Autodesk Inventor part; units mm, degrees
ref_plane "YZ Plane" through (0, 0, 0) normal (1, 0, 0) x (0, 1, 0)
ref_plane "XZ Plane" through (0, 0, 0) normal (0, 1, 0) x (-1, 0, 0)
ref_plane "XY Plane" through (0, 0, 0) normal (0, 0, 1) x (1, 0, 0)
sketch "Sketch1" plane through (0, 0, 0) normal (0, 1, 0) x (-1, 0, 0)
  line L0 (-15, 20.25) -> (15, 20.25)
  line L1 (15, 20.25) -> (15, -20.25)
  line L2 (15, -20.25) -> (-15, -20.25)
  line L3 (-15, -20.25) -> (-15, 20.25)
  line L4 (-15, 20.25) -> (15, -20.25) construction
  line L5 (15, 20.25) -> (-15, -20.25) construction
  point P0 (0, 0)
  dimension "d0" = 40.5
  dimension "d1" = 30
extrude "Plate1" add sketch "Sketch1" along normal blind 1.5
sketch "Sketch2" plane through (-15, 0, -21.75) normal (0, 0, 1) x (1, 0, 0)
  line L0 (30, 0) -> (0, 0)
  line L1 (0, 0) -> (0, 35.9)
  line L2 (0, 35.9) -> (30, 35.9)
  line L3 (30, 35.9) -> (30, 0)
edge flange "Flange1" height 35.9 angle 90 thickness 1.5 bend radius 0.31 thickness toward (0, 0, 1) relief tear relief width 1.5 relief depth 0.75 corner gap 0.31 corner form 0 edges at (0, 1.5, -20.25) (0, 1.5, 20.25) wall of the first edge with corners at (15, 0, -21.75) (-15, 0, -21.75) (-15, 35.9, -21.75) (15, 35.9, -21.75)
bend "Bend1"
corner "Corner1"
sketch "Sketch3" plane through (0, 1.5, 0) normal (0, 1, 0) x (1, 0, 0)
  circle A0 centre (7, 0) radius 0.7835
  circle A1 centre (0, -7) radius 0.7835
  circle A2 centre (-7, 0) radius 0.7835
  circle A3 centre (0, 7) radius 0.7835
  point P0 (0, 0)
hole "Hole1" at (0, 1.5, 7) at (7, 1.5, 0) at (-7, 1.5, 0) at (0, 1.5, -7) direction (0, -1, 0) diameter 2.1 depth 1.5
sketch "Sketch26" plane through (-15, 35.9, 21.75) normal (0, 0, 1) x (1, 0, 0)
  line L0 (30, 9.1) -> (25, 9.1)
  line L1 (25, 9.1) -> (25, -25.9)
  line L2 (25, -25.9) -> (30, -25.9)
  line L3 (30, -25.9) -> (30, 9.1)
  line L4 (0, 9.1) -> (5, 9.1)
  line L5 (5, 9.1) -> (5, -25.9)
  line L6 (5, -25.9) -> (0, -25.9)
  line L7 (0, -25.9) -> (0, 9.1)
  point P0 (15, -35.9)
  dimension "d91" = 35
  dimension "d92" = 5
  dimension "d93" = 10
  dimension "d94" = 10
  dimension "d95" = 5
  dimension "d96" = 35
  dimension "d97" = 10
  dimension "d98" = 10
extrude "Cut11" cut sketch "Sketch26" against normal blind 1.5
fillet "Corner Round1" radius 5 1 edges at (-15, 10, 21)
fillet "Corner Round2" radius 5 1 edges at (15, 10, 21)
mirror "Mirror1" about plane through (0, 0, 0) normal (0, 0, 1) of "Cut11"
fillet "Corner Round3" radius 5 1 edges at (-15, 10, -21)
fillet "Corner Round4" radius 5 1 edges at (15, 10, -21)
fillet "Corner Round5" radius 1 4 edges at (10, 35.9, -21) (10, 35.9, 21) (-10, 35.9, 21) (-10, 35.9, -21)
sketch "Sketch31" plane through (-15, 1.81, 21.75) normal (0, 0, 1) x (1, 0, 0)
  point P0 (15, -1.81)
sketch "Sketch34" plane through (0, 1.5, 0) normal (0, 1, 0) x (1, 0, 0)
  circle A0 centre (0, 0) radius 1.2295
  point P0 (0, 0)
hole "Hole13" at (0, 1.5, 0) direction (0, -1, 0) diameter 5.2 depth 1.5
sketch "Sketch35" plane through (-15, 1.81, 21.75) normal (0, 0, 1) x (1, 0, 0)
  circle A0 centre (15, 34.79) radius 2.925
  point P0 (15, -1.81)
hole "Hole16" at (0, 36.6, 21.75) direction (0, 0, -1) diameter 13.5 depth 1.5
sketch "Sketch36" plane through (15, 1.81, -21.75) normal (0, 0, -1) x (-1, 0, 0)
  circle A0 centre (15, 34.79) radius 4.48
  point P0 (15, -1.81)
hole "Hole17" at (0, 36.6, -21.75) direction (0, 0, 1) diameter 13.5 depth 1.5
sketch "Sketch37" plane through (-15, 1.81, 21.75) normal (0, 0, 1) x (1, 0, 0)
  circle A0 centre (23, 27.89) radius 0.7835
  circle A1 centre (22, 14.67) radius 0.7835
  circle A2 centre (15, 7.37) radius 0.7835
  circle A3 centre (8, 14.67) radius 0.7835
  circle A4 centre (7, 27.89) radius 0.7835
  point P0 (15, -1.81)
hole "Hole18" at (8, 29.7, 21.75) at (-8, 29.7, 21.75) at (7, 16.48, 21.75) at (-7, 16.48, 21.75) at (0, 9.18, 21.75) direction (0, 0, -1) diameter 2.1 depth 1.5
sketch "Sketch38" plane through (15, 1.81, -21.75) normal (0, 0, -1) x (-1, 0, 0)
  circle A0 centre (7.475, 7.19) radius 0.7835
  circle A1 centre (7.475, 22.29) radius 0.7835
  circle A2 centre (22.525, 7.19) radius 0.7835
  circle A3 centre (22.525, 22.29) radius 0.7835
  point P0 (15, -1.81)
hole "Hole19" at (7.525, 9, -21.75) at (7.525, 24.1, -21.75) at (-7.525, 9, -21.75) at (-7.525, 24.1, -21.75) direction (0, 0, 1) diameter 2.1 depth 1.5
equation "\"d18\" = Thickness"
equation "\"d99\" = Thickness"
equation "\"d143\" = Thickness"
equation "\"d164\" = Thickness"
equation "\"d171\" = Thickness"
equation "\"d178\" = Thickness"
equation "\"d185\" = Thickness"
equation "\"d2\" = Thickness"
equation "\"d3\" = BendReliefWidth"
equation "\"d4\" = BendReliefDepth"
equation "\"d5\" = MinimumRemnant"
equation "\"d6\" = TransitionRadius"
equation "\"d9\" = BendRadius"
equation "\"d10\" = CornerReliefSize"
equation "\"d11\" = GapSize"
equation "\"d12\" = JacobiRadiusSize"
equation "\"BendReliefWidth\" = Thickness"
equation "\"BendReliefDepth\" = 0.5 * Thickness"
equation "\"CornerReliefSize\" = 4 * Thickness"
equation "\"MinimumRemnant\" = 2 * Thickness"
equation "\"TransitionRadius\" = BendRadius"
equation "\"JacobiRadiusSize\" = BendRadius"
equation "\"GapSize\" = Thickness"
properties part number "axis_19_top_frame" material "Aluminum 6061-AHC"
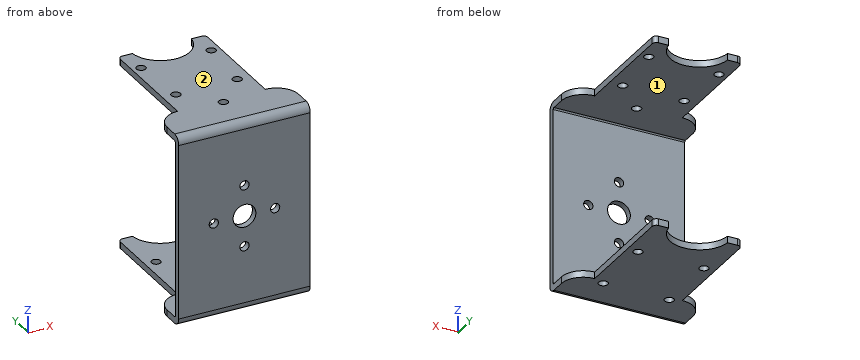
Could you check a few things on this model? Use its own coordinates, in mm. Face numbers are marked on the shaded views. A direction names the side the tool comes from. Coordinates: 2 decimals unless noted, no trailing zeros. Order: outer loops, then holes, each group sorted by start corner. A loop starts at its lowest first (then second) coordinate and runs counter-clockwise, first axis right, second up. Notation, with made-up numbers: M 29.5,9 L 65.5,9 A35 ccw 65.5,43 Z; hole C 14,26.25 d1. An arc over 180 degrees is marked long. Use a Markdown table: item, result. Add a question column.
Q1. Which directions (+Z, -Z, +X, -X, +Y, -Y) give clear straight access to the entire face, cutting with the end or side of a thin tool? Please do the marked faces 1 and 2.
Q2. I'm going to push flat-ended pins straight in: pin 1 (2.5 mm diameter, centred on x = -7, z = 0, fed in from +Y); pin 2 (1.9 mm diameter, centred on x = 0, z = -7, fed in from +Y); pin 3 (1.9 mm diameter, centred on x = 8, y = 29.7, fed in from +Z); pin 4 (3.5 mm diameter, centred on x = -8, y = 29.7, fed in from +Z). Where does each tip first touch, or does it pass through?
Q3. I want a section at A-A on y = 22. List the corners of the cut face in (x, z) for me, then the cut area to 3 significant figures.
Q4. If I drill on L1, parallel to X at y = 0.6, z = 0; L2, parallel to X at y = 16.48, z = 21.25; L3, parallel to X at y = 9, z = -21 (3 decimals), over which ranges is the centre line in solid material (lowest first)?
Q5. I want a section at B-B on z = -7. List the corners of the cut face in (x, y) for me, then the cut area to 4 significant figures.
Q6. I want a section at D-D on z = -0.5. List the corners of the cut face in (x, y) for me.
Q7. I want a section at C-C on y = 32. List the corners of the cut face in (x, z) for me.
Checked values:
| question | item | result |
|---|---|---|
| 1 | face 1 | +X, -X, +Y |
| 1 | face 2 | +Z, +X, -X, +Y, -Y |
| 2 | pin 1 | y = 1.5 |
| 2 | pin 2 | through |
| 2 | pin 3 | z = -20.25 |
| 2 | pin 4 | z = 21.75 |
| 3 | outline | M -10,-21.75 L 10,-21.75 L 10,-20.25 L -10,-20.25 Z; M -10,20.25 L 10,20.25 L 10,21.75 L -10,21.75 Z |
| 3 | area | 60.0 mm² |
| 4 | L1 | -15 to -8.05, -5.95 to -2.6, 2.6 to 5.95, 8.05 to 15 |
| 4 | L2 | -10 to -8.05, -5.95 to 5.95, 8.05 to 10 |
| 4 | L3 | -13 to -8.575, -6.475 to 6.475, 8.575 to 13 |
| 5 | outline | M -15,0 L -1.05,0 L -1.05,1.5 L -15,1.5 Z; M 1.05,0 L 15,0 L 15,1.5 L 1.05,1.5 Z |
| 5 | area | 41.85 mm² |
| 6 | outline | M -15,0 L -7.92,0 L -7.92,1.5 L -15,1.5 Z; M -6.08,0 L -2.55,0 L -2.55,1.5 L -6.08,1.5 Z; M 2.55,0 L 6.08,0 L 6.08,1.5 L 2.55,1.5 Z; M 7.92,0 L 15,0 L 15,1.5 L 7.92,1.5 Z |
| 7 | outline | M -10,-21.75 L -4.94,-21.75 L -4.94,-20.25 L -10,-20.25 Z; M -10,20.25 L -4.94,20.25 L -4.94,21.75 L -10,21.75 Z; M 4.94,-21.75 L 10,-21.75 L 10,-20.25 L 4.94,-20.25 Z; M 4.94,20.25 L 10,20.25 L 10,21.75 L 4.94,21.75 Z |
